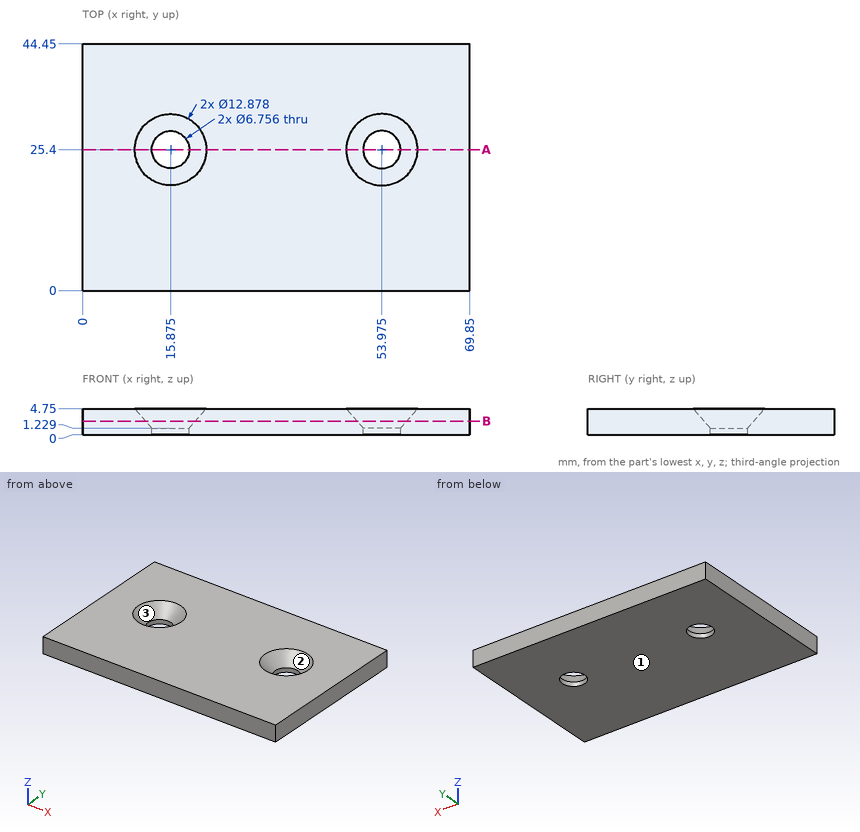
Design review of the part shown in the three views and the two pictorial views. Dimensions are in mm from the part's minimum x, y and z. Round coordinates to 2 decimals unless told otherwise and drop trailing zeros. Order: outer loops, then holes, each group sorted by start corner. A loop starts at its lowest first (then second) coordinate and runs counter-clockwise, first axis right, second up.
(1) Take a section at A-A, the plane y = 25.4. State the section outline as (x, z) points.
Working result:
outline: (0, 0) - (12.5, 0) - (12.5, 1.23) - (9.44, 4.75) - (0, 4.75) - close; (19.25, 0) - (50.6, 0) - (50.6, 1.23) - (47.54, 4.75) - (22.31, 4.75) - (19.25, 1.23) - close; (57.35, 0) - (69.85, 0) - (69.85, 4.75) - (60.41, 4.75) - (57.35, 1.23) - close
(2) Wall thickness on L1, parallel to X at y = 25.4, z = 0.8; L2, parallel to Y at x = 55.5, z = 2; L3, parallel to Y at x = 50.5, z = 4.45: over which ranges is each line inside the solid? List them lowest first.
Working result:
L1: x = 0 to 12.5, 19.25 to 50.6, 57.35 to 69.85
L2: y = 0 to 21.65, 29.15 to 44.45
L3: y = 0 to 20.29, 30.51 to 44.45
(3) Take a section at B-B, the plane z = 2.5. Count the separate pieces of the cut face and the enclosed holes in it, plus the area to 3 significant figures.
Working result:
separate pieces: 1
enclosed holes: 2
area: 2,980 mm2
(4) For P1, Ø6, axis at x = 53.975, y = 25.4, coming from the +Z side; P2, Ø1, axis at x = 12.5, y = 29, coming from the +Z side (1 decimal), all flat-tipped, find the tip position at first contact; note any pin that passes through.
Working result:
P1: passes through
P2: stops at z = 3.6
(5) Mouldability with a two-part tool opening along Y and no side actions: class the marked faces 1, 2 and 3 as released by +Y, released by -Y, zero draft, split by the parting line, or undercut.
Working result:
face 1: zero draft
face 2: undercut
face 3: undercut
